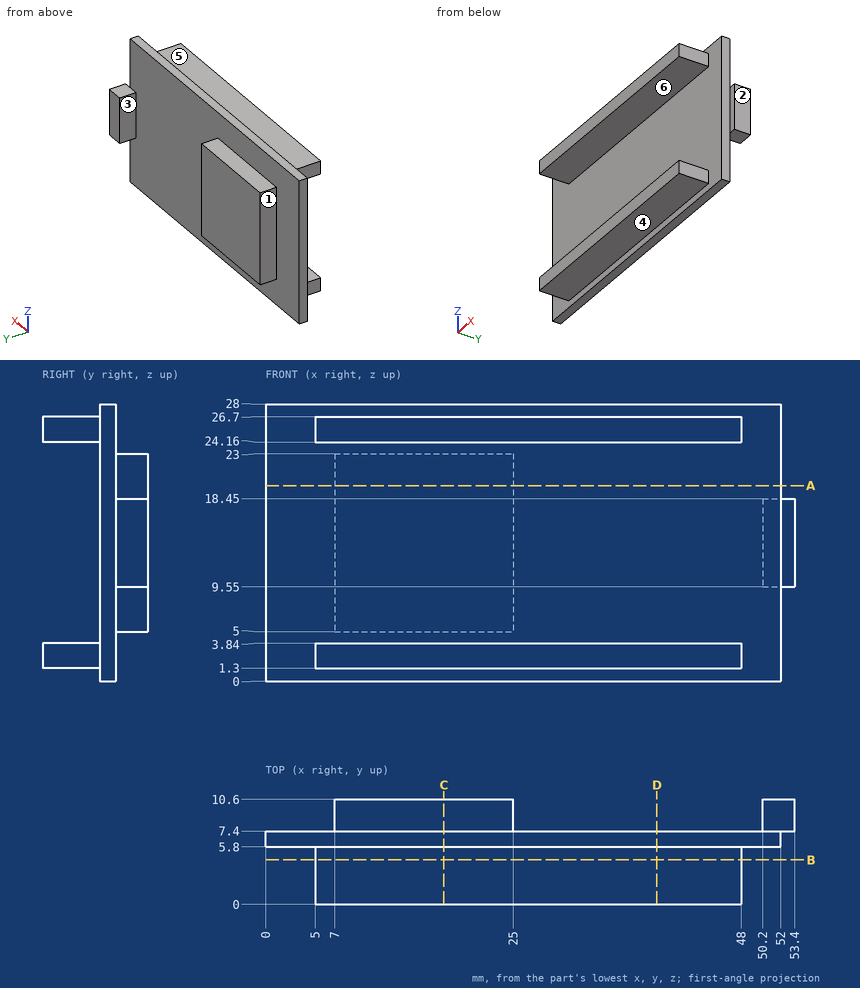
Here's the drawing with two shaded views (mm, measured from the low corner). I have some questions. A direction names the side the tool comes from. Round coordinates to 2 decimals unless told otherwise and drop trailing zeros. Order: outer loops, then holes, each group sorted by start corner. A loop starts at its lowest first (then second) coordinate and runs counter-clockwise, first axis right, second up. Notation, with made-up numbers: (-10, 11.25) -> (10, 11.25) arc R23 cw to (10, 28.25) -> close; hole circle Ø5 at (57, 55). An arc over 180 degrees is marked (long way). Write each question's results on one line, items separated by ' | '. Start each with the question number.
Item 1: If we section it at D-D, the plane x = 39.5: Write out the boundary of the cut face in (y, z), then the cut area to 3 significant figures.
Item 2: If we section it at C-C, the plane x = 18: Write out the boundary of the cut face in (y, z), then the cut area to 3 significant figures.
Item 3: If we section it at A-A, the plane z = 19.75: Write out the boundary of the cut face in (x, y).
Item 4: Thinking about a two-plate mould opening in Z: for the marked faces 4, 5 and 6, which applies, +Z half, -Z half, draft (parallel to the pull), parting line (faces both ways), or undercut?
Item 5: Which directions (+Z, -Z, +X, -X, +Y, -Y) give clear straight access to the entire face, cutting with the end or side of a thin tool? Please do the marked faces 1, 2 and 3.
Item 6: Please list where these lines run through material, in increasing order: L1, parallel to Z at x = 33, y = 0.75; L2, parallel to X at y = 8.75, z = 13; L3, parallel to Y at x = 32, z = 24.25.
Item 7: If we section it at B-B, the plane y = 4.5: Write out the boundary of the cut face in (x, z).
Item 8: Will these pins go through, and if not, where does the flat tip stop? pin 1 (3.5 mm diameter, centred on x = 51.5, y = 8.5, fed in from -Z); pin 2 (1 mm diameter, centred on y = 4, z = 20.5, fed in from +X); pin 3 (2 mm diameter, centred on y = 9.5, z = 21.5, fed in from +X); pin 4 (1.6 mm diameter, centred on y = 8.5, z = 16, fed in from -X).
Results:
1) outline: (0, 1.3) -> (5.8, 1.3) -> (5.8, 0) -> (7.4, 0) -> (7.4, 28) -> (5.8, 28) -> (5.8, 26.7) -> (0, 26.7) -> (0, 24.16) -> (5.8, 24.16) -> (5.8, 3.84) -> (0, 3.84) -> close | area: 74.3 mm2
2) outline: (0, 1.3) -> (5.8, 1.3) -> (5.8, 0) -> (7.4, 0) -> (7.4, 5) -> (10.6, 5) -> (10.6, 23) -> (7.4, 23) -> (7.4, 28) -> (5.8, 28) -> (5.8, 26.7) -> (0, 26.7) -> (0, 24.16) -> (5.8, 24.16) -> (5.8, 3.84) -> (0, 3.84) -> close | area: 132 mm2
3) outline: (0, 5.8) -> (52, 5.8) -> (52, 7.4) -> (25, 7.4) -> (25, 10.6) -> (7, 10.6) -> (7, 7.4) -> (0, 7.4) -> close
4) face 4: -Z half | face 5: +Z half | face 6: undercut
5) face 1: +Z, -Z, -X, +Y | face 2: +Z, -Z, +X, +Y, -Y | face 3: +Z, -Z, +Y
6) L1: z = 1.3 to 3.84, 24.16 to 26.7 | L2: x = 7 to 25, 50.2 to 53.4 | L3: y = 0 to 7.4
7) outline: (5, 1.3) -> (48, 1.3) -> (48, 3.84) -> (5, 3.84) -> close; (5, 24.16) -> (48, 24.16) -> (48, 26.7) -> (5, 26.7) -> close
8) pin 1: stops at z = 0 | pin 2: passes through | pin 3: stops at x = 25 | pin 4: stops at x = 7
